Here's how the part is built. I have some questions about the finished solid (model axes, mm). Face numbers are marked on the shaded views. A direction names the side the tool comes from. Round coordinates to 2 decimals unless told otherwise and drop trailing zeros. Write each loop counter-clockwise with the first axis right and the second up, starting at its lowest first coordinate (ties: lowest second). Pieces come first, ordered by that corner, then holes. Notation, with made-up numbers: M 73,49 L 130,49 A18 cw 130,57 Z; hole C 3,54.5 d6. An arc over 180 degrees is marked long. Use one line per item in the form item = value. Start each with the question number.
Q1. I need wall thicknesses on line 1 along Y through (x, z) = (4.45, 14.5); line 2 along X through (y, z) = (12, -9.5); line 3 along Y through (x, z) = (4.45, -8). Which ranges of each line are inside material? Lowest first, please. Write a range as from..to.
Q2. I want a section at A-A on x = 2.7. List the corners of the cut face in (y, z) for me, and give its area (3 significant figures).
Q3. I'm going to push flat-ended pins straight in: pin 1 Ø0.9 at (y, z) = (12, -8) entering from -X; pin 2 Ø2.5 at (x, z) = (4, -6.5) entering from -Y; pin 3 Ø0.6 at (x, z) = (0.5, 1) entering from +Y; pin 4 Ø1.7 at (x, z) = (2, 7) entering from +Y. Where does each tip first touch, or does it pass through?
Q4. I want a section at B-B on y = 13. List the corners of the cut face in (x, z) for me.
Q5. For the marked faces 1, 2, 3, 4 and 5, which set-ups out of +Z, -Z, +X, -X, +Y, -Y let a thin tool reach every point of the face, with its end or its side?
Q6. I want a section at C-C on z = 6. List the corners of the cut face in (x, y) for me, and give its area (3 significant figures).
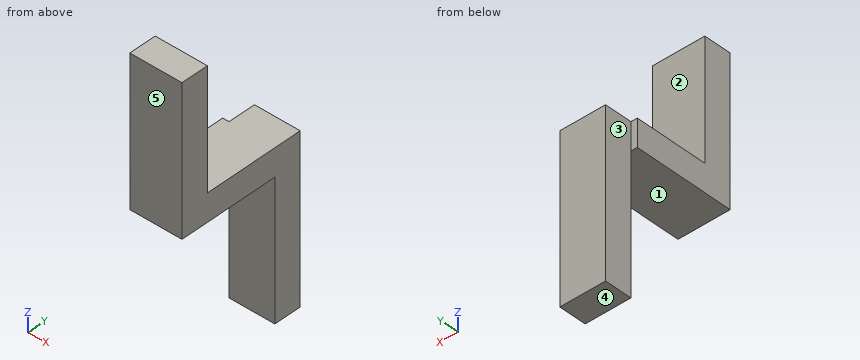
```python
from build123d import *

# Parameters (mm, degrees)
BOSS_EXTRUDE1_DEPTH = 5.7
SKETCH2_W           = 0.7
SKETCH2_H           = 3
CUT_EXTRUDE1_DEPTH  = 19


with BuildPart() as part:
    # Sketch1 → Boss-Extrude1 (new body)
    with BuildSketch(Plane(origin=(0, 0, 0), x_dir=(0, 0, -1), z_dir=(1, 0, 0))):
        Polygon((-16, 3), (-3, 3), (-3, 14), (15, 14), (15, 11), (0, 11), (0, 0), (-16, 0), align=None)
    extrude(amount=BOSS_EXTRUDE1_DEPTH)

    # Sketch2 → Cut-Extrude1 (cut, through all)
    with BuildSketch(Plane.XY.offset(3)):
        with Locations((0.35, 12.5)):
            Rectangle(SKETCH2_W, SKETCH2_H)
    extrude(amount=-CUT_EXTRUDE1_DEPTH, mode=Mode.SUBTRACT)


solid = part.part
```
Reported:
q1.line_1 = 0..3
q1.line_2 = 0.7..5.7
q1.line_3 = 11..14
q2.outline = M 0,0 L 11,0 L 11,-15 L 14,-15 L 14,3 L 3,3 L 3,16 L 0,16 Z
q2.area = 126 mm^2
q3.pin_1 = 0.7
q3.pin_2 = 11
q3.pin_3 = 14
q3.pin_4 = 3
q4.outline = M 0.7,-15 L 5.7,-15 L 5.7,3 L 0.7,3 Z
q5.face_1 = -Z, +X, -X, -Y
q5.face_2 = +Z, +X, -X, +Y
q5.face_3 = +Z, -Z, -X, +Y
q5.face_4 = -Z, +X, -X, +Y, -Y
q5.face_5 = +Z, -Z, +X, -X, -Y
q6.outline = M 0,0 L 5.7,0 L 5.7,3 L 0,3 Z
q6.area = 17.1 mm^2
